Here's how the part is built. I have some questions about the finished solid (model axes, mm). Face numbers are marked on the shaded views. Round coordinates to 2 decimals unless told otherwise and drop trailing zeros. Order: outer loops, then holes, each group sorted by start corner. A loop starts at its lowest first (then second) coordinate and runs counter-clockwise, first axis right, second up. Notation, with made-up numbers: (53, -26.75) - (108, -26.75) arc R18 cw to (108, -18.75) - close; hole circle Ø8 at (22, 24.25). An arc over 180 degrees is marked (long way). Answer as a JSON object with one key per item and string values.
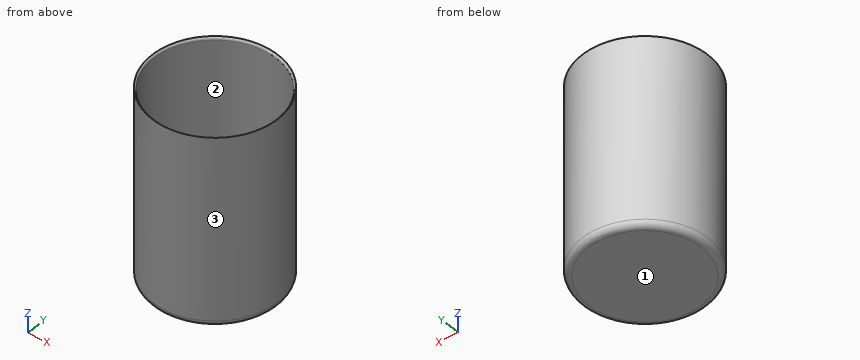
Autodesk Inventor part; units mm, degrees
ref_plane "YZ Plane" through (0, 0, 0) normal (1, 0, 0) x (0, 1, 0)
ref_plane "XZ Plane" through (0, 0, 0) normal (0, 1, 0) x (-1, 0, 0)
ref_plane "XY Plane" through (0, 0, 0) normal (0, 0, 1) x (1, 0, 0)
sketch "Sketch1" plane through (0, 0, 0) normal (0, 0, 1) x (1, 0, 0)
  circle A0 centre (0, 0) radius 40
  dimension "d0" = 80
extrude "Extrusion1" add sketch "Sketch1" along normal blind 120
sketch "Sketch2" plane through (0, 0, 120) normal (0, 0, 1) x (1, 0, 0)
  circle A0 centre (0, 0) radius 39
  dimension "d3" = 78
extrude "Extrusion2" cut sketch "Sketch2" against normal blind 118
fillet "Fillet1" radius 4 1 edges at (-40, 0, 0)
fillet "Fillet2" radius 2 1 edges at (-39, 0, 120)
properties part number "beaker1"
1. Imagine slicing it at A-A (y = 0). List the corners of the cut face in (x, z) for me, plus the area to 3 significant figures.
Responses:
{"outline": "(-40, 4) arc R4 ccw to (-36, 0) - (36, 0) arc R4 ccw to (40, 4) - (40, 120) arc R2 ccw to (39, 118.27) - (39, 2) - (-39, 2) - (-39, 118.27) arc R2 ccw to (-40, 120) - close", "area": "388 mm2"}
2. If I drill on L1, parallel to Y at x = 0, z = 43; L2, parallel to Z at x = -30.5, y = 13; L3, parallel to X at y = 2.5, z = 31, over which ranges is the centre line in solid material (lowest first)? Write a range as [from, to].
Responses:
{"L1": "[-40, -39], [39, 40]", "L2": "[0, 2]", "L3": "[-39.92, -38.92], [38.92, 39.92]"}
3. Thinking about a two-plate mould opening in X: for the marked faces 1, 2 and 3, which applies, pulls with the +X half, pulls with the -X half, needs draft (parallel to the pull), parting line crosses it, or undercut?
Responses:
{"face 1": "needs draft", "face 2": "undercut", "face 3": "parting line crosses it"}
4. Imagine slicing it at B-B (z = 25). List the corners of the cut face in (x, y) for me, plus the area to 3 significant figures.
Responses:
{"outline": "circle Ø80 at (0, 0); hole circle Ø78 at (0, 0)", "area": "248 mm2"}
5. For P1, Ø3, axis at x = 21, z = 65.5, coming from the +Y side; P2, Ø1.5, axis at x = 21, y = -8, coming from the +Z side; P3, Ø12, axis at x = -30.5, z = 106, coming from the +Y side, each with a flat end and sliding along its axis, tell me the tip position at first contact or that it passes through.
Responses:
{"P1": "y = 34.92", "P2": "z = 2", "P3": "y = 31.62"}
